Build history of the part. All positions in model axes, mm. Coordinates: 2 decimals unless noted, no trailing zeros. Write each loop counter-clockwise with the first axis right and the second up, starting at its lowest first coordinate (ties: lowest second). Pieces come first, ordered by that corner, then holes.
```python
from build123d import *

# Parameters (mm, degrees)
F0_W     = 655
F0_H     = 6
F0_W_2   = 25
F1_DEPTH = 50
F4_R     = 9.525
F5_DEPTH = 408
F6_R     = 9.525
F7_DEPTH = 408
F8_R     = 9.525
F9_DEPTH = 408


# Not quite as in the source:
# - a feature names something its author has since deleted; it is built from what else it names
# - the program builds the solid bodies; features that only make, move or delete a surface that nothing else refers to are left out


with BuildPart() as f1:
    # F0 (on Top) → F1 (new body)
    with BuildSketch(Plane.XY):
        Polygon((0, 1190), (0, 0), (680, 0), (705, 0), (705, 25), (705, 125), (705, 131), (705, 539), (705, 545), (705, 645), (705, 651), (705, 1059), (705, 1065), (705, 1165), (705, 1190), (680, 1190), align=None)
        Polygon((25, 1065), (25, 1165), (680, 1165), (680, 1065), (680, 1059), (680, 651), (680, 645), (680, 545), (680, 539), (680, 131), (680, 125), (680, 25), (25, 25), (25, 125), (25, 131), (25, 539), (25, 545), (25, 645), (25, 651), (25, 1059), align=None, mode=Mode.SUBTRACT)
        Polygon((705, 25), (705, 0), (1360, 0), (1385, 0), (2040, 0), (2065, 0), (2065, 25), (2065, 125), (2065, 131), (2065, 539), (2065, 545), (2065, 645), (2065, 651), (2065, 1059), (2065, 1065), (2065, 1165), (2065, 1190), (2040, 1190), (1385, 1190), (1360, 1190), (705, 1190), (705, 1165), (1360, 1165), (1385, 1165), (2040, 1165), (2040, 1065), (2040, 1059), (2040, 651), (2040, 645), (2040, 545), (2040, 539), (2040, 131), (2040, 125), (2040, 25), (1385, 25), (1360, 25), align=None)
        Polygon((2065, 25), (2065, 0), (2745, 0), (2745, 1190), (2065, 1190), (2065, 1165), (2720, 1165), (2720, 1065), (2720, 1059), (2720, 651), (2720, 645), (2720, 545), (2720, 539), (2720, 131), (2720, 125), (2720, 25), align=None)
        with Locations((352.5, 542)):
            Rectangle(F0_W, F0_H)
        with Locations((352.5, 128)):
            Rectangle(F0_W, F0_H)
        with Locations((352.5, 648)):
            Rectangle(F0_W, F0_H)
        with Locations((352.5, 1062)):
            Rectangle(F0_W, F0_H)
        with Locations((1032.5, 648)):
            Rectangle(F0_W, F0_H)
        with Locations((1712.5, 648)):
            Rectangle(F0_W, F0_H)
        with Locations((1712.5, 542)):
            Rectangle(F0_W, F0_H)
        with Locations((1032.5, 542)):
            Rectangle(F0_W, F0_H)
        with Locations((2392.5, 542)):
            Rectangle(F0_W, F0_H)
        with Locations((2392.5, 648)):
            Rectangle(F0_W, F0_H)
        with Locations((2392.5, 1062)):
            Rectangle(F0_W, F0_H)
        with Locations((1712.5, 1062)):
            Rectangle(F0_W, F0_H)
        with Locations((1032.5, 1062)):
            Rectangle(F0_W, F0_H)
        with Locations((2392.5, 128)):
            Rectangle(F0_W, F0_H)
        with Locations((1032.5, 128)):
            Rectangle(F0_W, F0_H)
        with Locations((1712.5, 128)):
            Rectangle(F0_W, F0_H)
        with Locations((1372.5, 128)):
            Rectangle(F0_W_2, F0_H)
        with Locations((1372.5, 542)):
            Rectangle(F0_W_2, F0_H)
        with Locations((1372.5, 1062)):
            Rectangle(F0_W_2, F0_H)
        with Locations((1372.5, 648)):
            Rectangle(F0_W_2, F0_H)
    extrude(amount=F1_DEPTH)

    # F4 (on face) → F5 (join, through all)
    with BuildSketch(Plane(origin=(0, 651, 0), x_dir=(-1, 0, 0), z_dir=(0, 1, 0))):
        with Locations((-156, 25)):
            Circle(F4_R)
        with Locations((-287, 25)):
            Circle(F4_R)
        with Locations((-418, 25)):
            Circle(F4_R)
        with Locations((-549, 25)):
            Circle(F4_R)
        with Locations((-2196, 25)):
            Circle(F4_R)
        with Locations((-2327, 25)):
            Circle(F4_R)
        with Locations((-2458, 25)):
            Circle(F4_R)
        with Locations((-2589, 25)):
            Circle(F4_R)
    extrude(amount=F5_DEPTH)

    # F6 (on face) → F7 (join, through all)
    with BuildSketch(Plane(origin=(0, 131, 0), x_dir=(-1, 0, 0), z_dir=(0, 1, 0))):
        with Locations((-838.5, 25)):
            Circle(F6_R)
        with Locations((-972, 25)):
            Circle(F6_R)
        with Locations((-1105.5, 25)):
            Circle(F6_R)
        with Locations((-1239, 25)):
            Circle(F6_R)
        with Locations((-1372.5, 25)):
            Circle(F6_R)
        with Locations((-1506, 25)):
            Circle(F6_R)
        with Locations((-1639.5, 25)):
            Circle(F6_R)
        with Locations((-1773, 25)):
            Circle(F6_R)
        with Locations((-1906.5, 25)):
            Circle(F6_R)
    extrude(amount=F7_DEPTH)

    # F8 (on face) → F9 (join, through all)
    with BuildSketch(Plane(origin=(0, 651, 0), x_dir=(-1, 0, 0), z_dir=(0, 1, 0))):
        with Locations((-838.5, 25)):
            Circle(F8_R)
        with Locations((-972, 25)):
            Circle(F8_R)
        with Locations((-1105.5, 25)):
            Circle(F8_R)
        with Locations((-1239, 25)):
            Circle(F8_R)
        with Locations((-1372.5, 25)):
            Circle(F8_R)
        with Locations((-1506, 25)):
            Circle(F8_R)
        with Locations((-1639.5, 25)):
            Circle(F8_R)
        with Locations((-1773, 25)):
            Circle(F8_R)
        with Locations((-1906.5, 25)):
            Circle(F8_R)
    extrude(amount=F9_DEPTH)


solid = f1.part
```
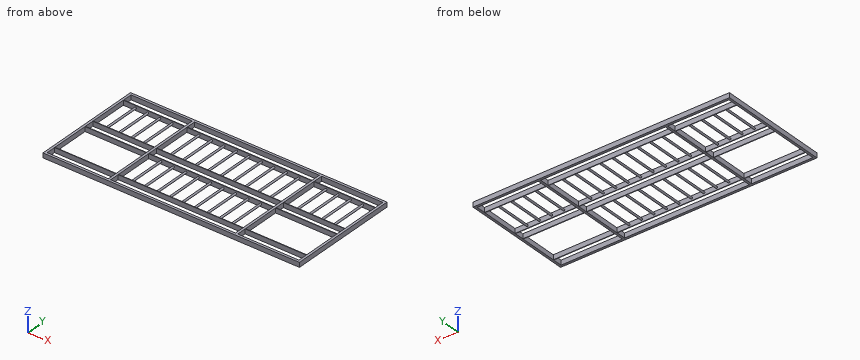
1. Flat gauge pin, fed straight in: pin 1 (25 mm diameter, centred on y = 839.5, z = 14, fed in from -X). Where does the tip first touch, or does it go through?
Computed values:
pin 1: stops at x = 0
2. Saw through at A-A on x = 1687. List the corners of the cut face in (y, z), plus the area to 3 significant figures.
Computed values:
outline: (0, 0) - (25, 0) - (25, 50) - (0, 50) - close; (125, 0) - (131, 0) - (131, 50) - (125, 50) - close; (539, 0) - (545, 0) - (545, 50) - (539, 50) - close; (645, 0) - (651, 0) - (651, 50) - (645, 50) - close; (1059, 0) - (1065, 0) - (1065, 50) - (1059, 50) - close; (1165, 0) - (1190, 0) - (1190, 50) - (1165, 50) - close
area: 3,700 mm2
3. Probe line 1 along Y through (x, z) = (1227, 22.5); line 2 along X through (y, z) = (382, 43); line 3 along Z through (x, y) = (417.5, 665). List the from-to ranges inside material, lowest first.
Computed values:
line 1: y = 0 to 25, 125 to 131, 539 to 545, 645 to 651, 1059 to 1065, 1165 to 1190
line 2: x = 0 to 25, 680 to 705, 2040 to 2065, 2720 to 2745
line 3: z = 15.49 to 34.51
4. Saw through at B-B on y = 511. State how many separate pieces and enclosed holes the cut face has, plus the area to 3 significant figures.
Computed values:
separate pieces: 13
enclosed holes: 0
area: 7,570 mm2
